```python
from build123d import *

# Parameters (mm, degrees)
ESTRUSIONE_ESTRUSIONE1_DEPTH                         = 50
SMUSSO1_SIZE                                         = 1.5
SMUSSO2_SIZE                                         = 5
FORO_LAMATO_PER_BULLONE_M5_A_TESTA_ESAGO_D           = 4.5
FORO_LAMATO_PER_BULLONE_M5_A_TESTA_ESAGO_DEPTH       = 70
FORO_LAMATO_PER_BULLONE_M5_A_TESTA_ESAGO_CBORE_D     = 10
FORO_LAMATO_PER_BULLONE_M5_A_TESTA_ESAGO_CBORE_DEPTH = 3
FORO_LAMATO_PER_BULLONE_M5_A_TESTA_ESAGO_TIP         = 1.351936393


with BuildPart() as part:
    # Schizzo1 → Estrusione-Estrusione1 (new body)
    with BuildSketch(Plane(origin=(0, 0, 0), x_dir=(0, 0, -1), z_dir=(1, 0, 0))):
        Polygon((-2.3, 0), (2.3, 0), (2.3, 2), (6.8, 2), (6.8, 8), (-6.8, 8), (-6.8, 2), (-2.3, 2), align=None)
    extrude(amount=ESTRUSIONE_ESTRUSIONE1_DEPTH)

    # Smusso1
    smusso1_edges = [part.edges().sort_by_distance(p)[0] for p in [
        (25, 8, 6.8),
        (25, 8, -6.8),
    ]]
    chamfer(smusso1_edges, length=SMUSSO1_SIZE)

    # Smusso2
    smusso2_edges = [part.edges().sort_by_distance(p)[0] for p in [
        (50, 8, 0),
        (0, 8, 0),
    ]]
    chamfer(smusso2_edges, length=SMUSSO2_SIZE)

    # Foro lamato per Bullone M5 a testa esagonale-1
    with Locations(Plane(origin=(0, 8, 0), x_dir=(1, 0, 0), z_dir=(0, 1, 0))):
        with Locations((15, 0), (35, 0)):
            CounterBoreHole(FORO_LAMATO_PER_BULLONE_M5_A_TESTA_ESAGO_D / 2, FORO_LAMATO_PER_BULLONE_M5_A_TESTA_ESAGO_CBORE_D / 2, FORO_LAMATO_PER_BULLONE_M5_A_TESTA_ESAGO_CBORE_DEPTH, depth=FORO_LAMATO_PER_BULLONE_M5_A_TESTA_ESAGO_DEPTH)
            with Locations((0, 0, -(FORO_LAMATO_PER_BULLONE_M5_A_TESTA_ESAGO_DEPTH + FORO_LAMATO_PER_BULLONE_M5_A_TESTA_ESAGO_TIP / 2))):  # 118° drill point
                Cone(0, FORO_LAMATO_PER_BULLONE_M5_A_TESTA_ESAGO_D / 2, FORO_LAMATO_PER_BULLONE_M5_A_TESTA_ESAGO_TIP, mode=Mode.SUBTRACT)


solid = part.part
```
For this review, take the finished solid that the model builds, in its own axes (mm). A direction names the side the tool comes from. Give positions to 0.01 mm unless a question says otherwise; leave off trailing zeros. Write each loop counter-clockwise with the first axis right and the second up, starting at its lowest first coordinate (ties: lowest second). Pieces come first, ordered by that corner, then holes. Notation, with made-up numbers: M -39,88.5 L -14,88.5 A18 ccw -14,95.5 Z; hole C 72.25,-26.5 d4. An arc over 180 degrees is marked long. One line per item, written item: value.
1) Take a section at A-A, the plane z = 0. Write out the cut boundary in (x, y).
Results are:
outline: M 0,0 L 12.75,0 L 12.75,5 L 10,5 L 10,8 L 5,8 L 0,3 Z; M 17.25,0 L 32.75,0 L 32.75,5 L 30,5 L 30,8 L 20,8 L 20,5 L 17.25,5 Z; M 37.25,0 L 50,0 L 50,3 L 45,8 L 40,8 L 40,5 L 37.25,5 Z
2) For faces 1 (the flat face through (25, 1, 2.3)), 2 (the cylindrical face through (30, 7, 0)), 3 (the flat face through (25, 2, -5)), list the 3-axis set-ups (+Z, -Z, +X, -X, +Y, -Y) from which the entire face can be reached by the end or side of a thin tool; tool diameter is ignored.
Results are:
face 1: +Z, +X, -X, -Y
face 2: +Y
face 3: -Z, +X, -X, -Y
3) The part is to be moulded in two halves that separate along Z. For faces 4 (the flat face through (25, 1, -2.3)), 5 (the flat face through (36, 5, 2.2)), 6 (the flat face through (25, 2, 5)), say which applies: +Z half, -Z half, draft (parallel to the pull), parting line (faces both ways), or undercut.
Results are:
face 4: -Z half
face 5: undercut
face 6: draft
4) For P1, Ø2, axis at x = 38.5, z = -3, coming from the -Y side; P2, Ø6, axis at x = 35, z = 0, coming from the +Y side; P3, Ø2, axis at x = 16.5, z = 4.5, coming from the -Y side; P4, Ø2.5, axis at x = 15, z = 0, coming from the +Y side, all flat-tipped, find the tip position at first contact; note any pin that passes through.
Results are:
P1: stops at y = 0
P2: stops at y = 5
P3: stops at y = 2
P4: passes through
5) Take a section at B-B, the plane y = 3.5. Write out the cut boundary in (x, z), then the cut area to 3 significant figures.
Results are:
outline: M 0.5,-6.8 L 49.5,-6.8 L 49.5,6.8 L 0.5,6.8 Z; hole C 15,0 d4.5; hole C 35,0 d4.5
area: 635 mm²
6) Take a section at D-D, the plane x = 44. Write out the cut boundary in (y, z).
Results are:
outline: M 0,-2.3 L 2,-2.3 L 2,-6.8 L 6.5,-6.8 L 8,-5.3 L 8,5.3 L 6.5,6.8 L 2,6.8 L 2,2.3 L 0,2.3 Z
7) For line 1 (X direction, y = 5.5, z = 0.5); line 2 (X direction, y = 5.75, z = -4.5); line 3 (Y direction, x = 18.5, z = -5), list the stretches that pass through material, from the lowest coordinate up. Write a range as from..to.
Results are:
line 1: x = 2.5..10.03, 19.97..30.03, 39.97..47.5
line 2: x = 2.75..12.82, 17.18..32.82, 37.18..47.25
line 3: y = 2..8
8) Take a section at C-C, the plane x = 15. Write out the cut boundary in (y, z).
Results are:
outline: M 0,-2.3 L 2,-2.3 L 2,-6.8 L 6.5,-6.8 L 8,-5.3 L 8,-5 L 5,-5 L 5,-2.25 L 0,-2.25 Z; M 0,2.25 L 5,2.25 L 5,5 L 8,5 L 8,5.3 L 6.5,6.8 L 2,6.8 L 2,2.3 L 0,2.3 Z
